CAD build for the part. Positions are in the model's coordinates, mm. A direction names the side the tool comes from. Round coordinates to 2 decimals unless told otherwise and drop trailing zeros. Loops run counter-clockwise (first coordinate to the right, second up) from the corner with the lowest first, then second, coordinate; pieces in that order, holes last. Notation, with made-up numbers: (-21, 49.5) -> (-5, 49.5) arc R26 ccw to (-5, 88.5) -> close; hole circle Ø9 at (69.25, 68). An arc over 180 degrees is marked (long way). Answer as CSV lines item,"result".
```python
from build123d import *

# Parameters (mm, degrees)
SKETCH1_W                = 38.1
SKETCH1_H                = 19.05
BOSS_EXTRUDE1_DEPTH      = 9.525
CUT_EXTRUDE1_DEPTH       = 10.525
CUT_EXTRUDE1_DEPTH_BACK  = 10.525
SKETCH3_R                = 1.984375
CUT_EXTRUDE2_DEPTH       = 10.525
CUT_EXTRUDE2_DEPTH_BACK  = 10.525
SKETCH4_W                = 3.175
SKETCH4_H                = 4.7625
SKETCH4_H_2              = 3.175
CUT_EXTRUDE3_DEPTH       = 20.05
CUT_EXTRUDE3_DEPTH_BACK  = 20.05
CUT_EXTRUDE9_START       = -2.38125
SKETCH11_R               = 3.683
CUT_EXTRUDE9_DEPTH       = 6.35
SKETCH12_W               = 6.35
SKETCH12_H               = 3.175
CUT_EXTRUDE10_DEPTH      = 10.525
CUT_EXTRUDE10_DEPTH_BACK = 10.525
SKETCH14_R               = 0.79375
CUT_EXTRUDE11_DEPTH      = 10.525
CUT_EXTRUDE11_DEPTH_BACK = 10.525
CUT_EXTRUDE12_DEPTH      = 4.7625
SKETCH16_W               = 3.175
SKETCH16_H               = 9.525
BOSS_EXTRUDE2_DEPTH      = 4.7625
SKETCH17_W               = 3.175
SKETCH17_H               = 9.525
BOSS_EXTRUDE3_DEPTH      = 4.7625
SKETCH18_R               = 0.7493
CUT_EXTRUDE13_DEPTH      = 29.943380657
SKETCH19_R               = 3.96875
BOSS_EXTRUDE4_DEPTH      = 1.778
SKETCH20_R               = 1.651
CUT_EXTRUDE14_DEPTH      = 21.828


with BuildPart() as part:
    # Sketch1 → Boss-Extrude1 (new body, symmetric)
    with BuildSketch(Plane(origin=(0, 0, 0), x_dir=(0, 0, -1), z_dir=(1, 0, 0))):
        Rectangle(SKETCH1_W, SKETCH1_H)
    extrude(amount=BOSS_EXTRUDE1_DEPTH, both=True)

    # Sketch2 → Cut-Extrude1 (cut, two sides)
    with BuildSketch(Plane(origin=(0, 0, 0), x_dir=(1, 0, 0), z_dir=(0, 1, 0))) as cut_extrude1_sk:
        with BuildLine():
            Line((91.748361933, -8.708899487), (9.525, 13.322783942))
            Line((9.525, 13.322783942), (3.066814498, 15.053249532))
            ThreePointArc((3.066814498, 15.053249532), (0, 19.05), (-3.066814498, 15.053249532))
            Line((-3.066814498, 15.053249532), (-9.525, 13.322783942))
            Line((-9.525, 13.322783942), (-91.748361933, -8.708899487))
            Line((-91.748361933, -8.708899487), (-91.748361933, 161.538876678))
            Line((-91.748361933, 161.538876678), (91.748361933, 161.538876678))
            Line((91.748361933, 161.538876678), (91.748361933, -8.708899487))
        make_face()
    extrude(amount=CUT_EXTRUDE1_DEPTH, mode=Mode.SUBTRACT)
    extrude(cut_extrude1_sk.sketch, amount=-CUT_EXTRUDE1_DEPTH_BACK, mode=Mode.SUBTRACT)

    # Sketch3 → Cut-Extrude2 (cut, two sides)
    with BuildSketch(Plane(origin=(0, 0, 0), x_dir=(1, 0, 0), z_dir=(0, 1, 0))) as cut_extrude2_sk:
        with Locations((0, 15.875)):
            Circle(SKETCH3_R)
    extrude(amount=CUT_EXTRUDE2_DEPTH, mode=Mode.SUBTRACT)
    extrude(cut_extrude2_sk.sketch, amount=-CUT_EXTRUDE2_DEPTH_BACK, mode=Mode.SUBTRACT)

    # Sketch4 → Cut-Extrude3 (cut, two sides)
    with BuildSketch(Plane.XY) as cut_extrude3_sk:
        with Locations((0, 7.14375)):
            Rectangle(SKETCH4_W, SKETCH4_H)
        with Locations((0, -7.9375)):
            Rectangle(SKETCH4_W, SKETCH4_H_2)
    extrude(amount=CUT_EXTRUDE3_DEPTH, mode=Mode.SUBTRACT)
    extrude(cut_extrude3_sk.sketch, amount=-CUT_EXTRUDE3_DEPTH_BACK, mode=Mode.SUBTRACT)

    # Sketch11 → Cut-Extrude9 (cut)
    with BuildSketch(Plane(origin=(0, 4.7625, 0), x_dir=(1, 0, 0), z_dir=(0, 1, 0)).offset(CUT_EXTRUDE9_START)):
        with Locations((0, 15.875)):
            Circle(SKETCH11_R)
    extrude(amount=-CUT_EXTRUDE9_DEPTH, mode=Mode.SUBTRACT)

    # Sketch12 → Cut-Extrude10 (cut, two sides)
    with BuildSketch(Plane(origin=(0, 0, 0), x_dir=(0, 0, -1), z_dir=(1, 0, 0))) as cut_extrude10_sk:
        with Locations((15.449630657, -7.9375)):
            Rectangle(SKETCH12_W, SKETCH12_H)
    extrude(amount=CUT_EXTRUDE10_DEPTH, mode=Mode.SUBTRACT)
    extrude(cut_extrude10_sk.sketch, amount=-CUT_EXTRUDE10_DEPTH_BACK, mode=Mode.SUBTRACT)

    # Sketch14 → Cut-Extrude11 (cut, two sides)
    with BuildSketch(Plane(origin=(0, 0, 0), x_dir=(0, 0, -1), z_dir=(1, 0, 0))) as cut_extrude11_sk:
        with Locations((-17.4625, -7.9375)):
            Circle(SKETCH14_R)
        with Locations((10.687130657, -7.9375)):
            Circle(SKETCH14_R)
    extrude(amount=CUT_EXTRUDE11_DEPTH, mode=Mode.SUBTRACT)
    extrude(cut_extrude11_sk.sketch, amount=-CUT_EXTRUDE11_DEPTH_BACK, mode=Mode.SUBTRACT)

    # Sketch15 → Cut-Extrude12 (cut)
    with BuildSketch(Plane(origin=(0, 9.525, 0), x_dir=(1, 0, 0), z_dir=(0, 1, 0))):
        Polygon((-9.525, 13.322783942), (-3.066814498, 15.053249532), (3.066814498, 15.053249532), (9.525, 13.322783942), (9.525, 19.05), (-9.525, 19.05), align=None)
    extrude(amount=-CUT_EXTRUDE12_DEPTH, mode=Mode.SUBTRACT)

    # Sketch16 → Boss-Extrude2 (add)
    with BuildSketch(Plane(origin=(9.525, 0, 0), x_dir=(0, 0, -1), z_dir=(1, 0, 0))):
        with Locations((8.305880657, -4.7625)):
            Rectangle(SKETCH16_W, SKETCH16_H)
    extrude(amount=BOSS_EXTRUDE2_DEPTH)

    # Sketch17 → Boss-Extrude3 (add)
    with BuildSketch(Plane.ZY.offset(9.525)):
        with Locations((-8.305880657, -4.7625)):
            Rectangle(SKETCH17_W, SKETCH17_H)
    extrude(amount=BOSS_EXTRUDE3_DEPTH)

    # Sketch18 → Cut-Extrude13 (cut, through all)
    with BuildSketch(Plane(origin=(0, 0, -9.893380657), x_dir=(-1, 0, 0), z_dir=(0, 0, -1))):
        with Locations((-11.90625, -4.7625)):
            Circle(SKETCH18_R)
        with Locations((11.90625, -4.7625)):
            Circle(SKETCH18_R)
    extrude(amount=-CUT_EXTRUDE13_DEPTH, mode=Mode.SUBTRACT)

    # Sketch19 → Boss-Extrude4 (add)
    with BuildSketch(Plane(origin=(0, 9.525, 0), x_dir=(1, 0, 0), z_dir=(0, 1, 0))):
        with Locations((-5.55625, 0.368380657)):
            Circle(SKETCH19_R)
        with Locations((5.55625, 0.368380657)):
            Circle(SKETCH19_R)
    extrude(amount=BOSS_EXTRUDE4_DEPTH)

    # Sketch20 → Cut-Extrude14 (cut, through all)
    with BuildSketch(Plane(origin=(0, 11.303, 0), x_dir=(1, 0, 0), z_dir=(0, 1, 0))):
        with Locations((-5.55625, 0.368380657)):
            Circle(SKETCH20_R)
        with Locations((5.55625, 0.368380657)):
            Circle(SKETCH20_R)
    extrude(amount=-CUT_EXTRUDE14_DEPTH, mode=Mode.SUBTRACT)


solid = part.part
```
Q1. Tool access for faces 1 (the flat face through (12, -6, -6.718)), 2 (the flat face through (-12, -6, -9.893)), 3 (the flat face through (1.588, -8, 3)), 4 (the flat face through (1, 4.762, -18)), 5 (the flat face through (-12, -6, -6.718)): list every direction of +Z, -Z, +X, -X, +Y, -Y with a clear straight run to the whole face (end or side of a thin tool).
Results:
face 1,"+Z, +X, +Y, -Y"
face 2,"-Z, -X, +Y, -Y"
face 3,"+Z, -Z, -Y"
face 4,"-Z, +X, -X, +Y"
face 5,"+Z, -X, +Y, -Y"
Q2. Drop flat-ended pins along their axis: pin 1 Ø10 at (y, z) = (7, -3.5) entering from +X (3 decimals); pin 2 Ø2.5 at (x, z) = (0.5, 1.5) entering from +Y (3 decimals); pin 3 Ø4 at (x, z) = (-5.56, -0.37) entering from -Y (3 decimals); pin 4 Ø1 at (x, z) = (12.5, -8.5) entering from +Y. Give the stop position or say it passes through.
Results:
pin 1,"x = 9.525"
pin 2,"y = 9.525"
pin 3,"y = -9.525"
pin 4,"y = 0"
Q3. Two-plate mould, pull along X, no slides. Class faces 6 (the flat face through (12, -6, -9.893)), 7 (the cylindrical face through (-9.52, 10.4, -0.54)), 8 (the flat face through (14.288, -5, -8)), 9 (the flat face through (1.588, 7, 2)): pulls with the +X half, pulls with the -X half, needs draft (parallel to the pull), parting line crosses it, or undercut.
Results:
face 6,"needs draft"
face 7,"undercut"
face 8,"pulls with the +X half"
face 9,"undercut"
Q4. Slice it at B-B, the plane x = 0. Give the cut face in (y, z), and give its area (3 significant figures).
Results:
outline,"(-6.35, -19.05) -> (-3.97, -19.05) -> (-3.97, -17.86) -> (-6.35, -17.86) -> close; (-6.35, -13.89) -> (-3.97, -13.89) -> (-3.97, -12.19) -> (2.38, -12.19) -> (2.38, -13.89) -> (4.76, -13.89) -> (4.76, 19.05) -> (-6.35, 19.05) -> close; (2.38, -19.05) -> (4.76, -19.05) -> (4.76, -17.86) -> (2.38, -17.86) -> close"
area,"361 mm2"
Q5. Slice it at A-A, the plane y = 5.5. Count the separate pieces of the cut face and the enclosed holes in it, and give its area (3 significant figures).
Results:
separate pieces,"2"
enclosed holes,"2"
area,"513 mm2"
Q6. Probe L1, parallel to Z at x = -2.25, y = -8; L2, parallel to X at y = -6, z = -6 (3 decimals); L3, parallel to Z at x = 2.75, y = 5.25. List the from-to ranges inside material, lowest first. Write a range as [from, to].
Results:
L1,"[-12.27, -11.48], [-9.9, 16.67], [18.25, 19.05]"
L2,"[-9.525, 9.525]"
L3,"[-15.05, 19.05]"
